from build123d import *

# Parameters (mm, degrees)
SKETCH_W           = 45
SKETCH_H           = 3
PAD_DEPTH          = 20
PAD001_DEPTH       = 45
SKETCH002_R        = 1.6
POCKET_DEPTH       = 4.561
SKETCH004_R        = 1.6
PAD002_DEPTH       = 45
PAD002_FACE9_R     = 1.6
POCKET001_DEPTH    = 10
POCKET001_FACE14_R = 1.6
POCKET002_DEPTH    = 10
SKETCH005_W        = 10
SKETCH005_H        = 8
POCKET003_DEPTH    = 20.001
SKETCH006_W        = 3
SKETCH006_H        = 5.26
POCKET004_DEPTH    = 45.001
CHAMFER_SIZE       = 2
SKETCH007_R        = 3
POCKET005_DEPTH    = 8.001


with BuildPart() as part:
    # Sketch → Pad (new body)
    with BuildSketch(Plane.XY):
        Rectangle(SKETCH_W, SKETCH_H)
    extrude(amount=PAD_DEPTH)

    # Sketch001 (on Face2 of Pad) → Pad001 (join)
    with BuildSketch(Plane.YZ.offset(22.5)):
        Polygon((1.5, 10), (1.5, 14.74), (3.06, 12.94), (3.06, 7.06), (1.5, 5.26), align=None)
    extrude(amount=-PAD001_DEPTH)

    # Sketch002 (on Face6 of Pad001) → Pocket (cut, through all)
    with BuildSketch(Plane.XZ.offset(1.5)):
        with Locations((-17.186, 10)):
            Circle(SKETCH002_R)
        with Locations((17.186, 10)):
            Circle(SKETCH002_R)
    extrude(amount=-POCKET_DEPTH, mode=Mode.SUBTRACT)

    # Sketch004 (on Face3 of Pocket) → Pad002 (join)
    with BuildSketch(Plane.YZ.offset(22.5)):
        with BuildLine():
            ThreePointArc((-5.5, 14), (-9.5, 10), (-5.5, 6))
            Line((-5.5, 6), (-1.5, 6))
            Line((-1.5, 14), (-1.5, 6))
            Line((-1.5, 14), (-5.5, 14))
        make_face()
        with Locations((-5.5, 10)):
            Circle(SKETCH004_R, mode=Mode.SUBTRACT)
    extrude(amount=-PAD002_DEPTH)

    # Pad002 Face9 → Pocket001 (cut)
    with BuildSketch(Plane(origin=(22.5, -5.065426, 10), x_dir=(0, -1, 0), z_dir=(1, 0, 0))):
        with BuildLine():
            ThreePointArc((0.434574, -4), (4.434574, 0), (0.434574, 4))
            Line((0.434574, 4), (-3.565426, 4))
            Line((-3.565426, 4), (-3.565426, -4))
            Line((-3.565426, -4), (0.434574, -4))
        make_face()
        with Locations((0.434574, 0)):
            Circle(PAD002_FACE9_R, mode=Mode.SUBTRACT)
    extrude(amount=-POCKET001_DEPTH, mode=Mode.SUBTRACT)

    # Pocket001 Face14 → Pocket002 (cut)
    with BuildSketch(Plane(origin=(-22.5, -5.065426, 10), x_dir=(0, 1, 0), z_dir=(-1, 0, 0))):
        with BuildLine():
            ThreePointArc((-0.434574, 4), (-4.434574, 0), (-0.434574, -4))
            Line((-0.434574, -4), (3.565426, -4))
            Line((3.565426, -4), (3.565426, 4))
            Line((3.565426, 4), (-0.434574, 4))
        make_face()
        with Locations((-0.434574, 0)):
            Circle(POCKET001_FACE14_R, mode=Mode.SUBTRACT)
    extrude(amount=-POCKET002_DEPTH, mode=Mode.SUBTRACT)

    # Sketch005 (on Face2 of Pocket002) → Pocket003 (cut, through all)
    with BuildSketch(Plane(origin=(0, 0, 0), x_dir=(1, 0, 0), z_dir=(0, 0, -1))):
        with Locations((0, 5.5)):
            Rectangle(SKETCH005_W, SKETCH005_H)
    extrude(amount=-POCKET003_DEPTH, mode=Mode.SUBTRACT)

    # Sketch006 (on Face5 of Pocket003) → Pocket004 (cut, through all)
    with BuildSketch(Plane(origin=(-22.5, 0, 0), x_dir=(0, -1, 0), z_dir=(-1, 0, 0))):
        with Locations((0, 17.37)):
            Rectangle(SKETCH006_W, SKETCH006_H)
        with Locations((0, 2.63)):
            Rectangle(SKETCH006_W, SKETCH006_H)
    extrude(amount=-POCKET004_DEPTH, mode=Mode.SUBTRACT)

    # Chamfer
    chamfer_edges = [part.edges().sort_by_distance(p)[0] for p in [
        (-12.5, -1.5, 10),
        (12.5, -1.5, 10),
    ]]
    chamfer(chamfer_edges, length=CHAMFER_SIZE)

    # Sketch007 (on Face29 of Chamfer) → Pocket005 (cut, through all)
    with BuildSketch(Plane.XZ.offset(1.5)):
        with Locations((-17.186, 10)):
            Circle(SKETCH007_R)
        with Locations((17.186, 10)):
            Circle(SKETCH007_R)
    extrude(amount=POCKET005_DEPTH, mode=Mode.SUBTRACT)


solid = part.part
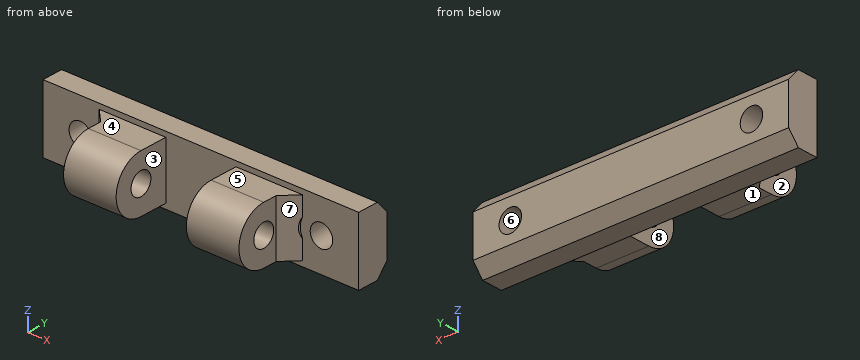
Source: CAD feature listing. Evaluate the final solid. Frame: model axes, mm. Face numbers are marked on the shaded views. A direction names the side the tool comes from. Coordinates: 2 decimals unless noted, no trailing zeros. Loops run counter-clockwise (first coordinate to the right, second up) from the corner with the lowest first, then second, coordinate; pieces in that order, holes last. Notation, with made-up numbers: M -22,-27 L -14,-27 A16 ccw -14,-12 Z; hole C 25.5,47 d3. An arc over 180 degrees is marked long. Answer in a Markdown table with one row per item.
Q1. Set-up query: the marked faces 1, 2, 3 and 4. Return all of +Z, -Z, +X, -X, +Y, -Y with unobstructed straight access to the full face (end or side cutting, diameter ignored); none if empty.
Answers below:
| item | result |
|---|---|
| face 1 | -Z, +X, -X, -Y |
| face 2 | +Z, -Z, -X, -Y |
| face 3 | +Z, -Z, -Y |
| face 4 | +Z, +X, -X, -Y |
Q2. Section C-C on z = 10. State how many separate pieces and enclosed holes the cut face has, plus the area to 3 significant figures.
Answers below:
| item | result |
|---|---|
| separate pieces | 5 |
| enclosed holes | 0 |
| area | 252 mm^2 |
Q3. Draft query along X for the marked faces 5, 6, 7 and 8. Return one class per face: pulls with the +X half, pulls with the -X half, needs draft (parallel to the pull), parting line crosses it, or undercut.
Answers below:
| item | result |
|---|---|
| face 5 | needs draft |
| face 6 | undercut |
| face 7 | pulls with the +X half |
| face 8 | undercut |
Q4. First-contact query: pin 1 (3 mm diameter, centred on y = -8, z = 10.5, fed in from -X); pin 2 (3 mm diameter, centred on x = 8.5, y = -4, fed in from -Z); pin 3 (5 mm diameter, centred on y = -5.5, z = 10, fed in from +X). Flat tips, straight axial feed; report the tip coordinate or a pass-through.
Answers below:
| item | result |
|---|---|
| pin 1 | stops at x = -12.5 |
| pin 2 | stops at z = 6 |
| pin 3 | stops at x = 13 |
Q5. Section B-B on x = -8.5. Return the cut outline in (y, z), plus the area to 3 significant figures.
Answers below:
| item | result |
|---|---|
| outline | M -5.5,6 L -1.5,6 L -1.5,5.26 L 1.5,5.26 L 3.06,7.06 L 3.06,12.94 L 1.5,14.74 L -1.5,14.74 L -1.5,14 L -5.5,14 A4 ccw Z; hole C -5.5,10 d3.2 |
| area | 89.5 mm^2 |
Q6. Ray query, probe 1 along Y at (x, z) = (8.5, 10); probe 2 along X at (y, z) = (-7.25, 8.25); probe 3 along X at (y, z) = (-0.5, 8.75). Return the intervals inside material, ascending. Write a range as from..to.
Answers below:
| item | result |
|---|---|
| probe 1 | y = -9.5..-7.1, -3.9..3.06 |
| probe 2 | x = -12.5..-5, 5..12.5 |
| probe 3 | x = -22.5..-18.18, -16.19..16.19, 18.18..22.5 |
Q7. Section A-A on y = -2.75. Return the cut outline in (x, z), plus the area to 3 significant figures.
Answers below:
| item | result |
|---|---|
| outline | M -13.25,6 L -5,6 L -5,14 L -13.25,14 Z; M 5,6 L 13.25,6 L 13.25,14 L 5,14 Z |
| area | 132 mm^2 |
Q8. Section D-D on y = 0.25. Return the cut outline in (x, z).
Answers below:
| item | result |
|---|---|
| outline | M -22.5,5.26 L 22.5,5.26 L 22.5,14.74 L -22.5,14.74 Z; hole C -17.19,10 d3.2; hole C 17.19,10 d3.2 |
